Source: CAD feature listing. Evaluate the final solid. Frame: model axes, mm. Face numbers are marked on the shaded views. A direction names the side the tool comes from. Give positions to 0.01 mm unless a question says otherwise; leave off trailing zeros. Order: outer loops, then holes, each group sorted by start corner. A loop starts at its lowest first (then second) coordinate and runs counter-clockwise, first axis right, second up.
from build123d import *

# Parameters (mm, degrees)
F0_W     = 52
F0_H     = 80
F1_DEPTH = 3
F2_W     = 52
F2_H     = 71
F3_DEPTH = 14
F4_R     = 4.5
F5_DEPTH = 10


with BuildPart() as f1:
    # F0 (on Top) → F1 (new body)
    with BuildSketch(Plane.XY):
        Rectangle(F0_W, F0_H)
    extrude(amount=F1_DEPTH)

    # F2 (on face) → F3 (join)
    with BuildSketch(Plane.XY.offset(3)):
        with Locations((0, -4.5)):
            Rectangle(F2_W, F2_H)
    extrude(amount=F3_DEPTH)

    # F4 (on face) → F5 (join)
    with BuildSketch(Plane(origin=(-26, 0, 0), x_dir=(0, -1, 0), z_dir=(-1, 0, 0))):
        with Locations((23.814216, 9.224292)):
            Circle(F4_R)
        with Locations((-18.612601, 7.083489)):
            Circle(F4_R)
    extrude(amount=F5_DEPTH)


solid = f1.part
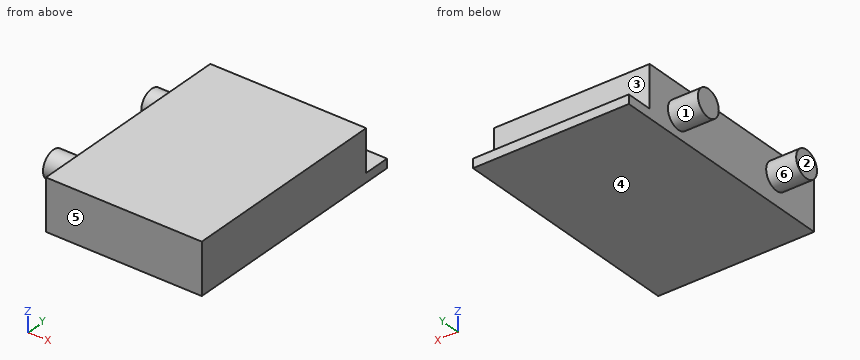
1) Section query C-C on x = -18.5. Output: boundary loops of the cut face in (y, z).
Checks:
outline: (-40, 0) - (40, 0) - (40, 3) - (31, 3) - (31, 17) - (-40, 17) - close
2) Section query B-B on y = -5. Output: boundary loops of the cut face in (x, z), and give its area (3 significant figures).
Checks:
outline: (-26, 0) - (26, 0) - (26, 17) - (-26, 17) - close
area: 884 mm2
3) First-contact query: pin 1 Ø8 at (y, z) = (22.5, 2) entering from -X; pin 2 Ø5 at (x, z) = (-17, 7.5) entering from +Y; pin 3 Ø4.5 at (x, y) = (-4, 34) entering from +Z. Flat tips, straight axial feed; report the tip coordinate or a pass-through.
Checks:
pin 1: stops at x = -36
pin 2: stops at y = 31
pin 3: stops at z = 3
4) Section query A-A on z = 8.25. Output: boundary loops of the cut face in (x, y).
Checks:
outline: (-36, -28.21) - (-26, -28.21) - (-26, -40) - (26, -40) - (26, 31) - (-26, 31) - (-26, 22.96) - (-36, 22.96) - (-36, 14.27) - (-26, 14.27) - (-26, -19.42) - (-36, -19.42) - close
5) Ray query, L1, parallel to Y at x = -9, z = 12; L2, parallel to X at y = -17, z = 3.5; L3, parallel to Z at x = 10, y = 37.5. Return the intervals inside material, ascending.
Checks:
L1: y = -40 to 31
L2: x = -26 to 26
L3: z = 0 to 3
6) Reachability of the marked faces 1 and 2 from +Z, -Z, +X, -X, +Y, -Y: full face, straight path, thin tool, end or side. Return the list, or none.
Checks:
face 1: -X
face 2: +Z, -Z, -X, +Y, -Y
7) Section query D-D on y = 16.5. Output: boundary loops of the cut face in (x, z), and give its area (3 significant figures).
Checks:
outline: (-36, 3.11) - (-26, 3.11) - (-26, 0) - (26, 0) - (26, 17) - (-26, 17) - (-26, 11.06) - (-36, 11.06) - close
area: 963 mm2
8) Pull-direction query (Y, two-part tool) for the marked faces 3, 4, 5 and 6; classes: +Y half, -Y half, draft (parallel to the pull), parting line (faces both ways), or undercut.
Checks:
face 3: +Y half
face 4: draft
face 5: -Y half
face 6: undercut
